Verification items for the finished model (mm, model axes). A direction names the side the tool comes from. Coordinates: 2 decimals unless noted, no trailing zeros. Write each loop counter-clockwise with the first axis right and the second up, starting at its lowest first coordinate (ties: lowest second). Pieces come first, ordered by that corner, then holes. Notation, with made-up numbers: (8, 67.5) -> (63, 67.5) arc R20 ccw to (63, 74.5) -> close; hole circle Ø5 at (-27.75, 21). An arc over 180 degrees is marked (long way). Answer in a Markdown table with one row per item.
```python
from build123d import *

# Parameters (mm, degrees)
BOSS_EXTRUDE2_DEPTH = 2.54
BOSS_EXTRUDE3_DEPTH = 15.24
SKETCH6_W           = 12.7
SKETCH6_H           = 6.35
CUT_EXTRUDE3_DEPTH  = 2.54


with BuildPart() as part:
    # Sketch1 → Boss-Extrude2 (new body)
    with BuildSketch(Plane.XY):
        with BuildLine():
            ThreePointArc((1.27, 97.858615874), (1.993851652, 99.606148348), (3.741384126, 100.33))
            Line((3.741384126, 100.33), (85.09, 100.33))
            ThreePointArc((85.09, 100.33), (86.886051224, 99.586051224), (87.63, 97.79))
            Line((87.63, 97.79), (87.63, 3.81))
            ThreePointArc((87.63, 3.81), (86.886051224, 2.013948776), (85.09, 1.27))
            Line((85.09, 1.27), (3.81, 1.27))
            ThreePointArc((3.81, 1.27), (2.013948776, 2.013948776), (1.27, 3.81))
            Line((1.27, 3.81), (1.27, 97.858615874))
        make_face()
    extrude(amount=BOSS_EXTRUDE2_DEPTH)

    # Sketch1<3> → Boss-Extrude3 (add)
    with BuildSketch(Plane.XY):
        with BuildLine():
            Line((0, 99.06), (0, 2.54))
            ThreePointArc((0, 2.54), (0.743948776, 0.743948776), (2.54, 0))
            Line((2.54, 0), (86.36, 0))
            ThreePointArc((86.36, 0), (88.156051224, 0.743948776), (88.9, 2.54))
            Line((88.9, 2.54), (88.9, 99.06))
            ThreePointArc((88.9, 99.06), (88.156051224, 100.856051224), (86.36, 101.6))
            Line((86.36, 101.6), (2.54, 101.6))
            ThreePointArc((2.54, 101.6), (0.743948776, 100.856051224), (0, 99.06))
        make_face()
        with BuildLine():
            Line((1.27, 97.858615874), (1.27, 3.81))
            ThreePointArc((1.27, 3.81), (2.013948776, 2.013948776), (3.81, 1.27))
            Line((3.81, 1.27), (85.09, 1.27))
            ThreePointArc((85.09, 1.27), (86.886051224, 2.013948776), (87.63, 3.81))
            Line((87.63, 3.81), (87.63, 97.79))
            ThreePointArc((87.63, 97.79), (86.886051224, 99.586051224), (85.09, 100.33))
            Line((85.09, 100.33), (3.741384126, 100.33))
            ThreePointArc((3.741384126, 100.33), (1.993851652, 99.606148348), (1.27, 97.858615874))
        make_face(mode=Mode.SUBTRACT)
    extrude(amount=BOSS_EXTRUDE3_DEPTH)

    # Sketch6 → Cut-Extrude3 (cut)
    with BuildSketch(Plane.XZ):
        with Locations((80.01, 12.065)):
            Rectangle(SKETCH6_W, SKETCH6_H)
    extrude(amount=-CUT_EXTRUDE3_DEPTH, mode=Mode.SUBTRACT)


solid = part.part
```
1. Section check A-A, the plane z = 5.5. Record the boundary of the cut face in (x, y), plus the area to 3 significant figures.
Geometry says:
| item | result |
|---|---|
| outline | (0, 2.54) arc R2.54 ccw to (2.54, 0) -> (86.36, 0) arc R2.54 ccw to (88.9, 2.54) -> (88.9, 99.06) arc R2.54 ccw to (86.36, 101.6) -> (2.54, 101.6) arc R2.54 ccw to (0, 99.06) -> close; hole (1.27, 3.81) arc R2.54 ccw to (3.81, 1.27) -> (85.09, 1.27) arc R2.54 ccw to (87.63, 3.81) -> (87.63, 97.79) arc R2.54 ccw to (85.09, 100.33) -> (3.74, 100.33) arc R2.47 ccw to (1.27, 97.86) -> close |
| area | 477 mm^2 |
2. Section check D-D, the plane z = 11.25. Record the boundary of the cut face in (x, y), plus the area to 3 significant figures.
Geometry says:
| item | result |
|---|---|
| outline | (0, 2.54) arc R2.54 ccw to (2.54, 0) -> (73.66, 0) -> (73.66, 1.27) -> (3.81, 1.27) arc R2.54 cw to (1.27, 3.81) -> (1.27, 97.86) arc R2.47 cw to (3.74, 100.33) -> (85.09, 100.33) arc R2.54 cw to (87.63, 97.79) -> (87.63, 3.81) arc R2.54 cw to (86.36, 1.61) -> (86.36, 0) arc R2.54 ccw to (88.9, 2.54) -> (88.9, 99.06) arc R2.54 ccw to (86.36, 101.6) -> (2.54, 101.6) arc R2.54 ccw to (0, 99.06) -> close |
| area | 461 mm^2 |
3. Tool access check on faces 1 (the cylindrical face through (86.906, 99.566, 8.801)), 2 (the flat face through (0, 51, 8)). Record the directions out of +Z, -Z, +X, -X, +Y, -Y that give a thin tool (end or side, any length) a straight path to the whole face; none if there is none.
Geometry says:
| item | result |
|---|---|
| face 1 | +Z |
| face 2 | +Z, -Z, -X, +Y, -Y |
4. Section check B-B, the plane y = 11.5. Record the boundary of the cut face in (x, z).
Geometry says:
| item | result |
|---|---|
| outline | (0, 0) -> (88.9, 0) -> (88.9, 15.24) -> (87.63, 15.24) -> (87.63, 2.54) -> (1.27, 2.54) -> (1.27, 15.24) -> (0, 15.24) -> close |
5. Mould release check, pull along X, two halves, no side actions. Record for faces 3 (the flat face through (44, 52, 0)), 4 (the cylindrical face through (88, 101, 8)), 5 (the flat face through (44, 1.27, 9)), 6 (the cylindrical face through (0.764, 100.876, 7.513)): released by +X, released by -X, zero draft, split by the parting line, or undercut.
Geometry says:
| item | result |
|---|---|
| face 3 | zero draft |
| face 4 | released by +X |
| face 5 | undercut |
| face 6 | released by -X |
6. Thickness scan on line 1 (Y direction, x = 15, z = 6); line 2 (X direction, y = 7.5, z = 6.75); line 3 (Z direction, x = 5, y = 5.5). Record the ranges inside material, lowest first. Write a range as from..to.
Geometry says:
| item | result |
|---|---|
| line 1 | 0..1.27, 100.33..101.6 |
| line 2 | 0..1.27, 87.63..88.9 |
| line 3 | 0..2.54 |
7. Section check C-C, the plane x = 59. Record the boundary of the cut face in (y, z).
Geometry says:
| item | result |
|---|---|
| outline | (0, 0) -> (101.6, 0) -> (101.6, 15.24) -> (100.33, 15.24) -> (100.33, 2.54) -> (1.27, 2.54) -> (1.27, 15.24) -> (0, 15.24) -> close |
8. Depth check by flat-ended pin: P1, Ø12, axis at x = 55, y = 48.5, coming from the +Z side; P2, Ø0.8, axis at y = 1, z = 12.5, coming from the -X side; P3, Ø0.6, axis at y = 0.5, z = 11.5, coming from the +X side. Enter the tip coordinate at first touch or a pass-through.
Geometry says:
| item | result |
|---|---|
| P1 | z = 2.54 |
| P2 | x = 0.27 |
| P3 | x = 88.21 |
